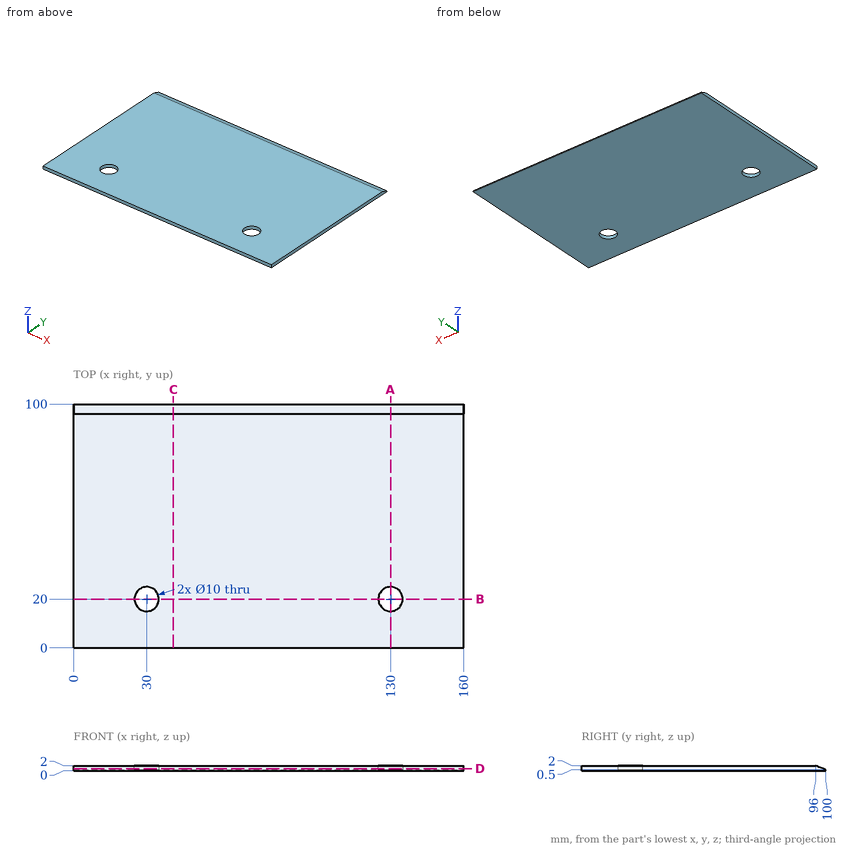
The drawing under review shows one solid part. Ordinate dimensions are in mm from its lowest x, y, z. Coordinates: 2 decimals unless noted, no trailing zeros. Order: outer loops, then holes, each group sorted by start corner. A loop starts at its lowest first (then second) coordinate and runs counter-clockwise, first axis right, second up. Notation, with made-up numbers: M 64.5,-6 L 119.5,-6 A13 ccw 119.5,5 Z; hole C 48,81.5 d3. An arc over 180 degrees is marked long. Use a Markdown table: item, result.
(1) Add section C-C (x = 41). Give the boundary of the cut face in (y, z), then the cut area to 3 significant figures.
Worked answers:
| item | result |
|---|---|
| outline | M 0,0 L 100,0 L 100,0.5 L 96,2 L 0,2 Z |
| area | 197 mm2 |
(2) Add section B-B (y = 20). Give the boundary of the cut face in (x, z).
Worked answers:
| item | result |
|---|---|
| outline | M 0,0 L 25,0 L 25,2 L 0,2 Z; M 35,0 L 125,0 L 125,2 L 35,2 Z; M 135,0 L 160,0 L 160,2 L 135,2 Z |
(3) Add section A-A (x = 130). Give the boundary of the cut face in (y, z).
Worked answers:
| item | result |
|---|---|
| outline | M 0,0 L 15,0 L 15,2 L 0,2 Z; M 25,0 L 100,0 L 100,0.5 L 96,2 L 25,2 Z |
(4) Add section D-D (z = 0.85). Give the boundary of the cut face in (x, y), then the cut area to 3 significant figures.
Worked answers:
| item | result |
|---|---|
| outline | M 0,0 L 160,0 L 160,99.07 L 0,99.07 Z; hole C 30,20 d10; hole C 130,20 d10 |
| area | 15,700 mm2 |
(5) Wall thickness on probe 1 along Y at (x, z) = (30, 0.45); probe 2 along X at (y, z) = (23, 1.75): over which ranges is each line inside the solid? List them lowest first.
Worked answers:
| item | result |
|---|---|
| probe 1 | y = 0 to 15, 25 to 100 |
| probe 2 | x = 0 to 26, 34 to 126, 134 to 160 |
